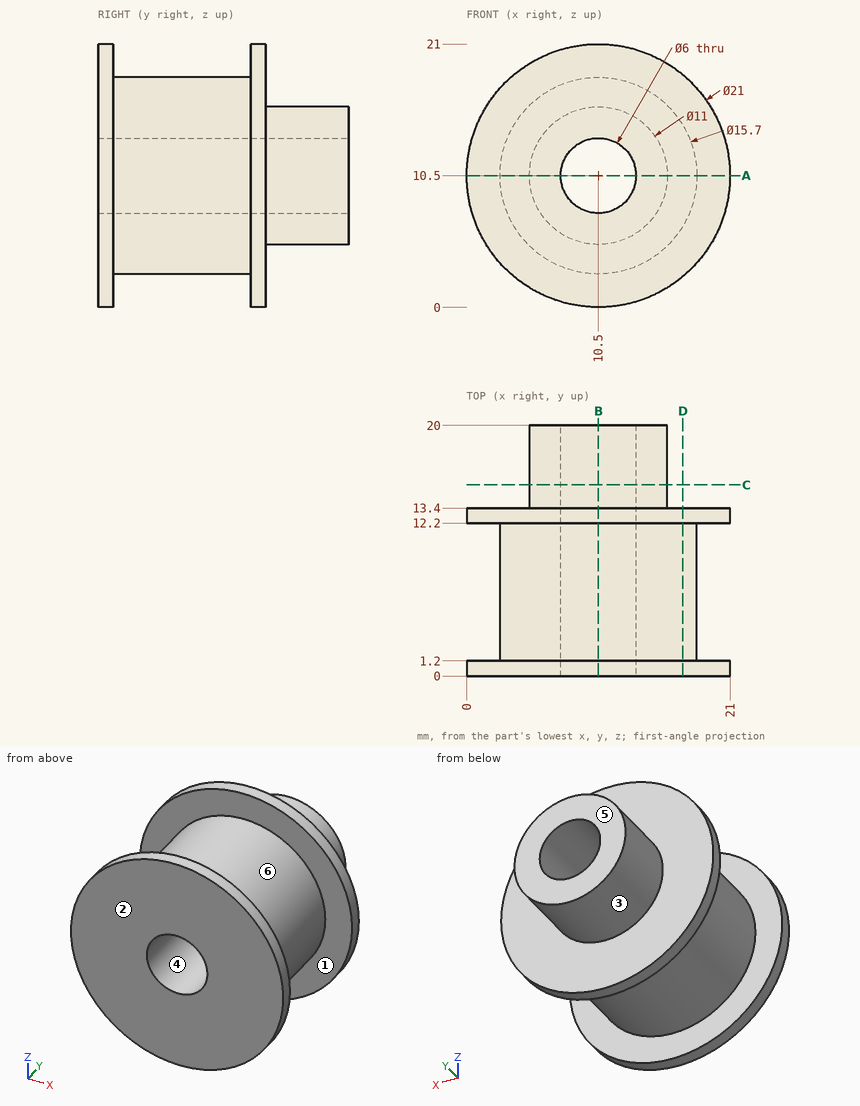
Could you check a few things on this drawing? It's one solid part, dimensions in mm from its lowest x, y, z. A direction names the side the tool comes from. Give positions to 0.01 mm unless a question says otherwise; leave off trailing zeros. Order: outer loops, then holes, each group sorted by start corner. A loop starts at its lowest first (then second) coordinate and runs counter-clockwise, first axis right, second up. Notation, with made-up numbers: (73, -27.5) - (100, -27.5) arc R5 cw to (100, -22.5) - close; hole circle Ø6 at (10, 0.5). An arc over 180 degrees is marked (long way). One line per question, with ' | ' between items. Start each with the question number.
Item 1: I want a section at D-D on x = 17.25. Write out the boundary of the cut face in (y, z).
Item 2: I need wall thicknesses on probe 1 along X at (y, z) = (5.5, 10.5); probe 2 along Y at (x, z) = (6, 3). Which ranges of each line are inside material? Lowest first, please. Write a range as [from, to].
Item 3: I want a section at A-A on z = 10.5. Write out the boundary of the cut face in (x, y).
Item 4: For the marked faces 1, 2 and 3, which set-ups out of +Z, -Z, +X, -X, +Y, -Y let a thin tool reach every point of the face, with its end or its side?
Item 5: I want a section at C-C on y = 15.25. Write out the boundary of the cut face in (x, z), then the cut area to 3 significant figures.
Item 6: Thinking about a two-plate mould opening in Z: for the marked faces 4, 5 and 6, which applies, pulls with the +Z half, pulls with the -Z half, needs draft (parallel to the pull), parting line crosses it, or undercut?
Item 7: I'm going to push flat-ended pins straight in: pin 1 Ø3.5 at (x, z) = (10.5, 10.5) entering from +Y; pin 2 Ø1.5 at (x, z) = (17, 13) entering from +Y; pin 3 Ø1.5 at (x, y) = (12, 6) entering from +Z; pin 4 Ø12 at (y, z) = (16.5, 17) entering from -X. Where does each tip first touch, or does it pass through?
Item 8: I want a section at B-B on x = 10.5. Write out the boundary of the cut face in (y, z).
Verdict:
1) outline: (0, 2.46) - (1.2, 2.46) - (1.2, 6.49) - (12.2, 6.49) - (12.2, 2.46) - (13.4, 2.46) - (13.4, 18.54) - (12.2, 18.54) - (12.2, 14.51) - (1.2, 14.51) - (1.2, 18.54) - (0, 18.54) - close
2) probe 1: [2.65, 7.5], [13.5, 18.35] | probe 2: [0, 1.2], [12.2, 13.4]
3) outline: (0, 0) - (7.5, 0) - (7.5, 20) - (5, 20) - (5, 13.4) - (0, 13.4) - (0, 12.2) - (2.65, 12.2) - (2.65, 1.2) - (0, 1.2) - close; (13.5, 0) - (21, 0) - (21, 1.2) - (18.35, 1.2) - (18.35, 12.2) - (21, 12.2) - (21, 13.4) - (16, 13.4) - (16, 20) - (13.5, 20) - close
4) face 1: none | face 2: +Z, -Z, +X, -X, -Y | face 3: +Y
5) outline: circle Ø11 at (10.5, 10.5); hole circle Ø6 at (10.5, 10.5) | area: 66.8 mm^2
6) face 4: undercut | face 5: needs draft | face 6: parting line crosses it
7) pin 1: through | pin 2: y = 13.4 | pin 3: z = 18.31 | pin 4: x = 0.09
8) outline: (0, 0) - (1.2, 0) - (1.2, 2.65) - (12.2, 2.65) - (12.2, 0) - (13.4, 0) - (13.4, 5) - (20, 5) - (20, 7.5) - (0, 7.5) - close; (0, 13.5) - (20, 13.5) - (20, 16) - (13.4, 16) - (13.4, 21) - (12.2, 21) - (12.2, 18.35) - (1.2, 18.35) - (1.2, 21) - (0, 21) - close
